The model under review builds one solid part; all positions refer to its coordinate system, in mm. Round coordinates to 2 decimals unless told otherwise and drop trailing zeros. Write each loop counter-clockwise with the first axis right and the second up, starting at its lowest first coordinate (ties: lowest second). Pieces come first, ordered by that corner, then holes. Notation, with made-up numbers: (85, -11.75) -> (109, -11.75) arc R4 ccw to (109, -4.75) -> close; hole circle Ø10 at (50.5, -39.5). An arc over 180 degrees is marked (long way). Answer as a JSON object with one key per item and string values. Group by question number.
1) We need section A-A, the plane y = 121. Write out the cut boundary in (x, z).
2) To check wall thickness, follow probe 1 along X at (y, z) = (293.5, 1.1); probe 2 along X at (y, z) = (384.5, -0.6); probe 3 along X at (y, z) = (58.5, -0.35). State the ranges of each line that lie inside material, in increasing order. Write a range as [from, to].
3) Insertion check: pin 1 Ø1.5 at (y, z) = (333.5, 1) entering from +X; pin 2 Ø0.6 at (x, z) = (248, 1) entering from +Y. Each pin has a flat end and moves straight along its axis. Give the tip position at first contact, or say it passes through.
4) We need section C-C, the plane x = 20. Write out the cut boundary in (y, z), then the cut area to 3 significant figures.
5) We need section B-B, the plane z = 0.35. Write out the cut boundary in (x, y), then the cut area to 3 significant figures.
from build123d import *

# Parameters (mm, degrees)
LINEAR_AUSTRAGEN_D_NN1_DEPTH = 2.5


with BuildPart() as part:
    # Skizze1 → Linear-Austragen-Dünn1 (new, symmetric)
    with BuildSketch(Plane.XY):
        with BuildLine():
            Line((247.5, 300), (247.5, 0))
            ThreePointArc((247.5, 0), (245.303300859, -5.303300859), (240, -7.5))
            Line((240, -7.5), (-240, -7.5))
            ThreePointArc((-240, -7.5), (-245.303300859, -5.303300859), (-247.5, 0))
            Line((-247.5, 0), (-247.5, 440))
            ThreePointArc((-247.5, 440), (-240, 447.5), (-232.5, 440))
            Line((-232.5, 440), (-232.5, 275))
            ThreePointArc((-232.5, 275), (-225.612554872, 265.496737288), (-214.437599567, 269.084114669))
            Line((-214.437599567, 269.084114669), (-214.840719588, 269.379908935))
            ThreePointArc((-214.840719588, 269.379908935), (-225.456927129, 265.971900424), (-232, 275))
            Line((-232, 275), (-232, 440))
            ThreePointArc((-232, 440), (-240, 448), (-248, 440))
            Line((-248, 440), (-248, 0))
            ThreePointArc((-248, 0), (-245.656854249, -5.656854249), (-240, -8))
            Line((-240, -8), (240, -8))
            ThreePointArc((240, -8), (245.656854249, -5.656854249), (248, 0))
            Line((248, 0), (248, 300))
            Line((248, 300), (247.5, 300))
        make_face()
    extrude(amount=LINEAR_AUSTRAGEN_D_NN1_DEPTH, both=True)


solid = part.part
Here are the results:
{
 "1": {"outline": "(-248, -2.5) -> (-247.5, -2.5) -> (-247.5, 2.5) -> (-248, 2.5) -> close; (247.5, -2.5) -> (248, -2.5) -> (248, 2.5) -> (247.5, 2.5) -> close"},
 "2": {"probe 1": "x = [-248, -247.5], [-232.5, -232], [247.5, 248]", "probe 2": "x = [-248, -247.5], [-232.5, -232]", "probe 3": "x = [-248, -247.5], [247.5, 248]"},
 "3": {"pin 1": "stops at x = -232", "pin 2": "stops at y = 300"},
 "4": {"outline": "(-8, -2.5) -> (-7.5, -2.5) -> (-7.5, 2.5) -> (-8, 2.5) -> close", "area": "2.50 mm^2"},
 "5": {"outline": "(-248, 0) arc R8 ccw to (-240, -8) -> (240, -8) arc R8 ccw to (248, 0) -> (248, 300) -> (247.5, 300) -> (247.5, 0) arc R7.5 cw to (240, -7.5) -> (-240, -7.5) arc R7.5 cw to (-247.5, 0) -> (-247.5, 440) arc R7.5 cw to (-232.5, 440) -> (-232.5, 275) arc R10 ccw to (-214.44, 269.08) -> (-214.84, 269.38) arc R9.5 cw to (-232, 275) -> (-232, 440) arc R8 ccw to (-248, 440) -> close", "area": "729 mm^2"}
}
